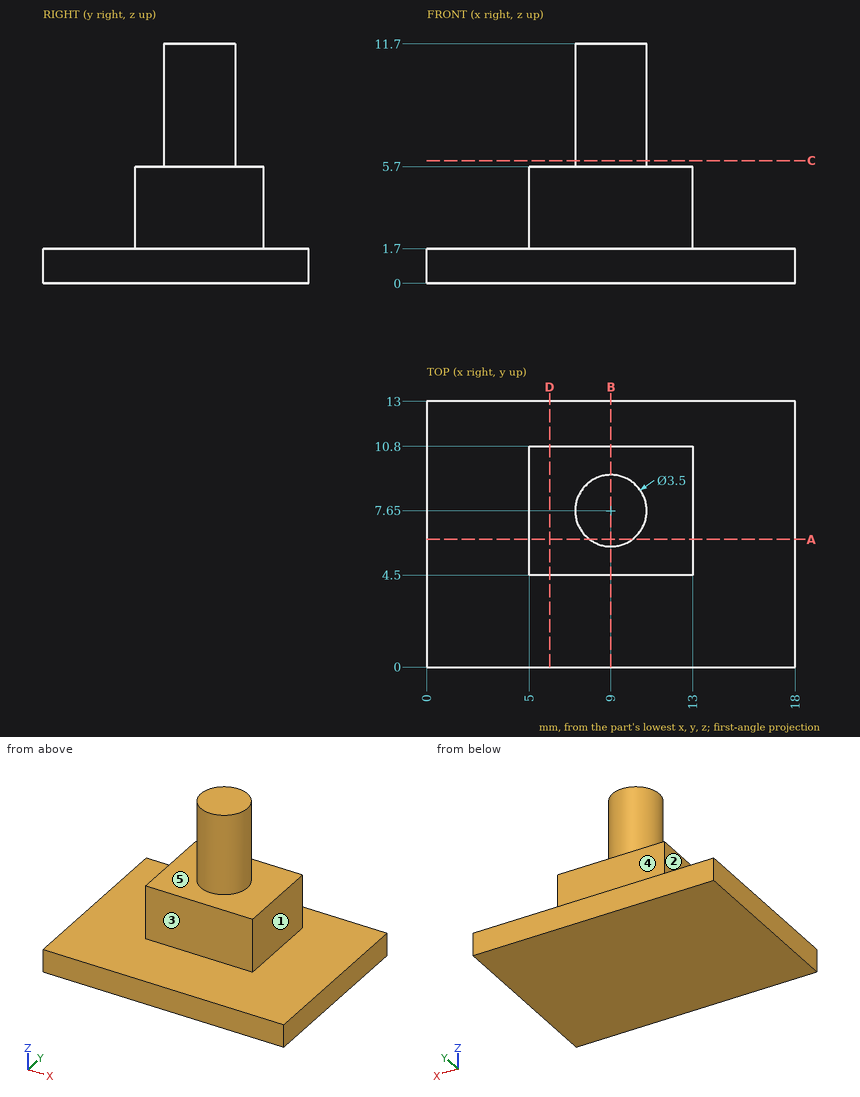
Study the drawing (mm; zero at the part's minimum x, y, z) and answer. A direction names the side the tool comes from. Round coordinates to 2 decimals unless told otherwise and drop trailing zeros. Write each loop counter-clockwise with the first axis right and the second up, starting at its lowest first coordinate (ties: lowest second). Pieces come first, ordered by that corner, then holes. Notation, with made-up numbers: (31, 85) - (76, 85) arc R13 cw to (76, 105) - close; hole circle Ø6 at (-11.5, 43). An arc over 180 degrees is marked (long way). Use a Markdown table: item, result. Add a question column.
1. The part is cut by section B-B (x = 9). Write down the section's boundary in (y, z).
2. The part is cut by section A-A (y = 6.25). Write down the section's boundary in (x, z), and give its area (3 significant figures).
3. Flat-ended cylindrical pins translate along their axes: P1, Ø3, axis at y = 5.5, z = 2.5, coming from the +X side; P2, Ø1.2, axis at y = 7.5, z = 4.5, coming from the -X side; P3, Ø3, axis at x = 15, y = 9, coming from the +Z side; P4, Ø2, axis at y = 8.5, z = 4, coming from the +X side. Find the tip coordinate at first contact, or state that the pin passes through.
4. The part is cut by section D-D (x = 6). Write down the section's boundary in (y, z), and give its area (3 significant figures).
5. The part is cut by section C-C (z = 6). Write down the section's boundary in (x, y), and give its area (3 significant figures).
6. Consider line 1 (Z direction, x = 1.5, y = 7.75); line 2 (Z direction, x = 6, y = 5.25); line 3 (Y direction, x = 7.75, z = 3.5). Determine where each line is inside the solid, lowest interval first.
7. A tool of negligible diameter and unlimited length cuts with its end or side. For the marked faces 1, 2, 3, 4 and 5, from which of +Z, -Z, +X, -X, +Y, -Y can it reach the whole face along a straight path? Write none if from no direction.
Reported:
| question | item | result |
|---|---|---|
| 1 | outline | (0, 0) - (13, 0) - (13, 1.7) - (10.8, 1.7) - (10.8, 5.7) - (9.4, 5.7) - (9.4, 11.7) - (5.9, 11.7) - (5.9, 5.7) - (4.5, 5.7) - (4.5, 1.7) - (0, 1.7) - close |
| 2 | outline | (0, 0) - (18, 0) - (18, 1.7) - (13, 1.7) - (13, 5.7) - (10.05, 5.7) - (10.05, 11.7) - (7.95, 11.7) - (7.95, 5.7) - (5, 5.7) - (5, 1.7) - (0, 1.7) - close |
| 2 | area | 75.2 mm^2 |
| 3 | P1 | x = 18 |
| 3 | P2 | x = 5 |
| 3 | P3 | z = 1.7 |
| 3 | P4 | x = 13 |
| 4 | outline | (0, 0) - (13, 0) - (13, 1.7) - (10.8, 1.7) - (10.8, 5.7) - (4.5, 5.7) - (4.5, 1.7) - (0, 1.7) - close |
| 4 | area | 47.3 mm^2 |
| 5 | outline | circle Ø3.5 at (9, 7.65) |
| 5 | area | 9.62 mm^2 |
| 6 | line 1 | 0 to 1.7 |
| 6 | line 2 | 0 to 5.7 |
| 6 | line 3 | 4.5 to 10.8 |
| 7 | face 1 | +Z, +X, +Y, -Y |
| 7 | face 2 | +Z, -X, +Y, -Y |
| 7 | face 3 | +Z, +X, -X, -Y |
| 7 | face 4 | +Z, +X, -X, +Y |
| 7 | face 5 | +Z |
